Can you work these out from the drawing? Everything is in mm from the part's minimum corner. Round coordinates to 2 decimals unless told otherwise and drop trailing zeros. Loops run counter-clockwise (first coordinate to the right, second up) from the corner with the lowest first, then second, coordinate; pieces in that order, holes last. Notation, with made-up numbers: (30.25, -7.5) -> (62.25, -7.5) arc R24 cw to (62.25, 24.5) -> close; hole circle Ø10 at (36.25, -18). An arc over 180 degrees is marked (long way). Answer as a JSON object with one key per item and string values.
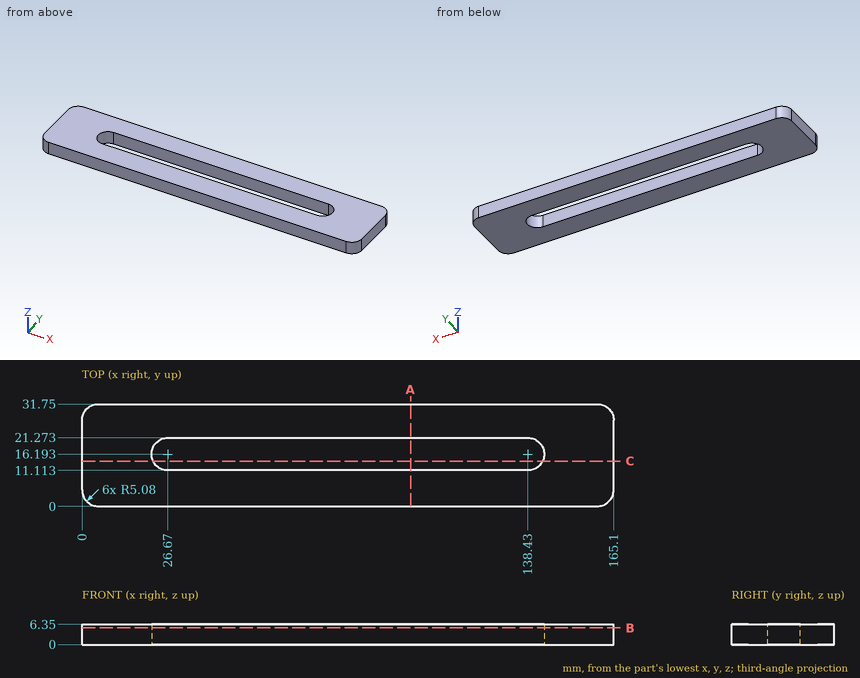
Q1. I want a section at B-B, the plane z = 5.25. Write out the boundary of the cut face in (x, y).
Determined:
{"outline": "(0, 5.08) arc R5.08 ccw to (5.08, 0) -> (160.02, 0) arc R5.08 ccw to (165.1, 5.08) -> (165.1, 26.67) arc R5.08 ccw to (160.02, 31.75) -> (5.08, 31.75) arc R5.08 ccw to (0, 26.67) -> close; hole (26.67, 11.11) -> (138.43, 11.11) arc R5.08 ccw to (138.43, 21.27) -> (26.67, 21.27) arc R5.08 ccw to start"}
Q2. If I drill on L1, parallel to Y at x = 36.5, z = 0.5; L2, parallel to X at y = 16.5, z = 1; L3, parallel to X at y = 12, z = 3.5 (1 decimal), over which ranges is the centre line in solid material (lowest first)? Write a range as [from, to].
Determined:
{"L1": "[0, 11.11], [21.27, 31.75]", "L2": "[0, 21.6], [143.5, 165.1]", "L3": "[0, 23.8], [141.3, 165.1]"}
Q3. I want a section at C-C, the plane y = 14. Write out the boundary of the cut face in (x, z).
Determined:
{"outline": "(0, 0) -> (22.09, 0) -> (22.09, 6.35) -> (0, 6.35) -> close; (143.01, 0) -> (165.1, 0) -> (165.1, 6.35) -> (143.01, 6.35) -> close"}
Q4. I want a section at A-A, the plane x = 102. Write out the boundary of the cut face in (y, z), then the cut area to 3 significant figures.
Determined:
{"outline": "(0, 0) -> (11.11, 0) -> (11.11, 6.35) -> (0, 6.35) -> close; (21.27, 0) -> (31.75, 0) -> (31.75, 6.35) -> (21.27, 6.35) -> close", "area": "137 mm²"}
